Source: CAD feature listing. Evaluate the final solid. Frame: model axes, mm. Face numbers are marked on the shaded views. A direction names the side the tool comes from. Round coordinates to 2 decimals unless told otherwise and drop trailing zeros. Write each loop counter-clockwise with the first axis right and the second up, starting at its lowest first coordinate (ties: lowest second). Pieces come first, ordered by that corner, then holes. Notation, with made-up numbers: M -34.75,64.5 L -8.75,64.5 A20 ccw -8.75,76.5 Z; hole C 52,29 d11. An arc over 180 degrees is marked long. Answer in a Markdown table with one row per item.
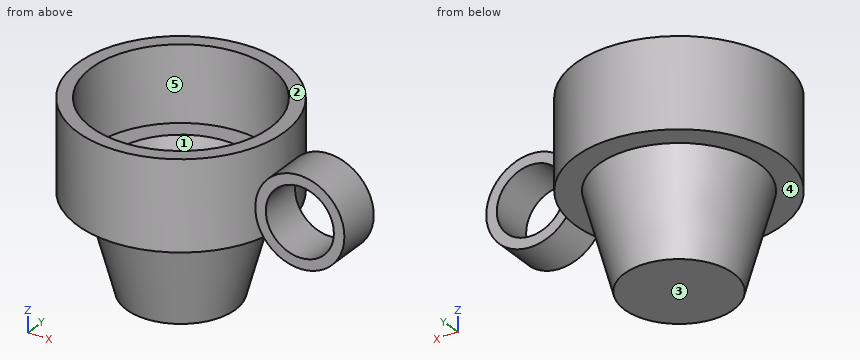
from build123d import *

# Parameters (mm, degrees)
F2_R     = 25.470351
F2_R_2   = 19.454516
F3_DEPTH = 25


with BuildPart() as f1:
    # F0 (on Front) → F1 (revolve)
    with BuildSketch(Plane.XZ):
        Polygon((25.09743, -41.101545), (0, -41.101545), (0, -49.096275), (31.210871, -49.096275), (46.123819, 5.827051), (59.280757, 5.827051), (59.280757, 56.741983), (51.286027, 56.741983), (51.286027, 13.821781), (40.010378, 13.821781), align=None)
    revolve(axis=Axis((0, 0, -45.09891), (0, 0, -1)))

    # F2 (on Front) → F3 (join)
    with BuildSketch(Plane.XZ):
        with Locations((84.688164, 27.397014)):
            Circle(F2_R)
        with Locations((84.688164, 27.397014)):
            Circle(F2_R_2, mode=Mode.SUBTRACT)
    extrude(amount=F3_DEPTH)


solid = f1.part
Q1. Contact query for flat-ended pins moving along their axis: pin 1 Ø25 at (x, y) = (3.5, -3.5) entering from +Z; pin 2 Ø8 at (y, z) = (16.5, 36.5) entering from +X; pin 3 Ø1.5 at (x, z) = (6, 21) entering from +Y. Output: stop coordinate, or through.
Solutions:
| item | result |
|---|---|
| pin 1 | stops at z = -41.1 |
| pin 2 | stops at x = 57.95 |
| pin 3 | stops at y = 59.05 |
Q2. Material intervals for probe 1 along Y at (x, z) = (0, 24.5); probe 2 along Z at (x, y) = (53, 2); probe 3 along Y at (x, z) = (36.5, 43.5), sorted ascending.
Solutions:
| item | result |
|---|---|
| probe 1 | y = -59.28 to -51.29, 51.29 to 59.28 |
| probe 2 | z = 5.83 to 56.74 |
| probe 3 | y = -46.71 to -36.03, 36.03 to 46.71 |
Q3. Pull-direction query (X, two-part tool) for the marked faces 1 and 2; classes: pulls with the +X half, pulls with the -X half, needs draft (parallel to the pull), parting line crosses it, or undercut.
Solutions:
| item | result |
|---|---|
| face 1 | undercut |
| face 2 | needs draft |
Q4. Section B-B (z = 37.5). Return loops of the section in (x, y).
Solutions:
| item | result |
|---|---|
| outline | C 0,0 d118.56; M 61.31,-25 L 68.06,-25 L 68.06,0 L 61.31,0 Z; M 101.31,-25 L 108.07,-25 L 108.07,0 L 101.31,0 Z; hole C 0,0 d102.57 |
Q5. Section A-A (x = 93.5). Return loops of the section in (y, z), and give its area (3 significant figures).
Solutions:
| item | result |
|---|---|
| outline | M -25,3.5 L 0,3.5 L 0,10.05 L -25,10.05 Z; M -25,44.74 L 0,44.74 L 0,51.29 L -25,51.29 Z |
| area | 328 mm2 |
Q6. Section D-D (z = -37). Return loops of the section in (x, y).
Solutions:
| item | result |
|---|---|
| outline | C 0,0 d68.99; hole C 0,0 d52.42 |
Q7. Access query for the marked faces 3, 4 and 5. Directions: +Z, -Z, +X, -X, +Y, -Y. A direction counts if a zero-diameter tool reaches every point of the face in a straight line with its end or side. Return the directions, or none.
Solutions:
| item | result |
|---|---|
| face 3 | -Z, +X, -X, +Y, -Y |
| face 4 | -Z |
| face 5 | +Z |
Q8. Section C-C (x = 0). Return loops of the section in (y, z), and give its area (3 significant figures).
Solutions:
| item | result |
|---|---|
| outline | M -59.28,5.83 L -46.12,5.83 L -31.21,-49.1 L 31.21,-49.1 L 46.12,5.83 L 59.28,5.83 L 59.28,56.74 L 51.29,56.74 L 51.29,13.82 L 40.01,13.82 L 25.1,-41.1 L -25.1,-41.1 L -40.01,13.82 L -51.29,13.82 L -51.29,56.74 L -59.28,56.74 Z |
| area | 2,310 mm2 |
